Answer from the drawing. Dimensions are ordinates in mm from the lowest x, y and z of the part. Coordinates: 2 decimals unless noted, no trailing zeros. Order: outer loops, then holes, each group sorted by start corner. A loop starts at its lowest first (then second) coordinate and runs counter-clockwise, first axis right, second up. Notation, with made-up numbers: (-21.75, 30.25) - (-13.75, 30.25) arc R21 ccw to (-13.75, 63.25) - close; hole circle Ø6 at (18.25, 2). An arc over 180 degrees is marked (long way). Use a Markdown table: item, result. Add a question column.
Item 1: The part is cut by section A-A, the plane z = 2.5. Give the vertices of the cut face in (x, y), then the cut area to 3 significant figures.
Item 2: Find the intervals of material crossed by line 1 along X through (y, z) = (0.5, 2.6); line 2 along X through (y, z) = (2.6, 1.8); line 3 along Z through (x, y) = (3, 2.35), in increasing order.
Item 3: The part is cut by section C-C, the plane y = 1.65. Give the vertices of the cut face in (x, z).
Item 4: The part is cut by section D-D, the plane x = 20. Give the vertices of the cut face in (y, z), then the cut area to 3 significant figures.
Item 5: The mould has two halves that part along Z. Classify the marked faces 1, 2 and 3: released by +Z, released by -Z, zero draft, split by the parting line, or undercut.
Item 6: The part is cut by section B-B, the plane x = 3. Give the vertices of the cut face in (y, z).
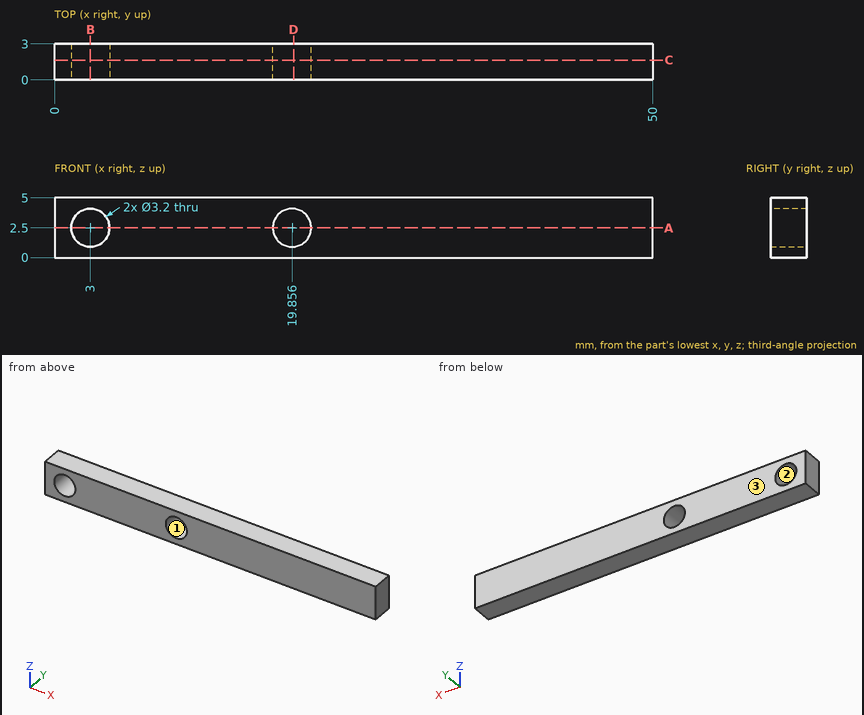
Solution:
| question | item | result |
|---|---|---|
| 1 | outline | (0, 0) - (1.4, 0) - (1.4, 3) - (0, 3) - close; (4.6, 0) - (18.26, 0) - (18.26, 3) - (4.6, 3) - close; (21.46, 0) - (50, 0) - (50, 3) - (21.46, 3) - close |
| 1 | area | 131 mm2 |
| 2 | line 1 | x = 0 to 1.4, 4.6 to 18.26, 21.45 to 50 |
| 2 | line 2 | x = 0 to 1.56, 4.44 to 18.42, 21.29 to 50 |
| 2 | line 3 | z = 0 to 0.9, 4.1 to 5 |
| 3 | outline | (0, 0) - (50, 0) - (50, 5) - (0, 5) - close; hole circle Ø3.2 at (3, 2.5); hole circle Ø3.2 at (19.86, 2.5) |
| 4 | outline | (0, 0) - (3, 0) - (3, 0.91) - (0, 0.91) - close; (0, 4.09) - (3, 4.09) - (3, 5) - (0, 5) - close |
| 4 | area | 5.44 mm2 |
| 5 | face 1 | undercut |
| 5 | face 2 | undercut |
| 5 | face 3 | zero draft |
| 6 | outline | (0, 0) - (3, 0) - (3, 0.9) - (0, 0.9) - close; (0, 4.1) - (3, 4.1) - (3, 5) - (0, 5) - close |
